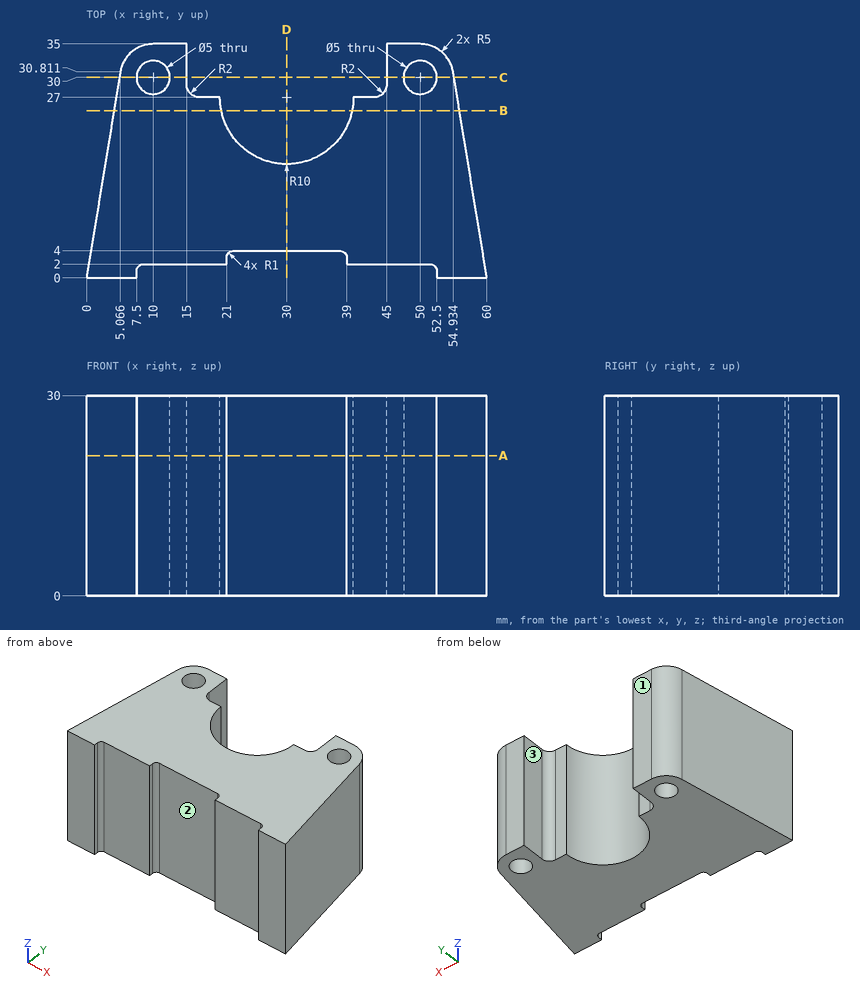
Job drawing, mm, ordinate dimensions from the low corner. One solid piece. A direction names the side the tool comes from. Round coordinates to 2 decimals unless told otherwise and drop trailing zeros. Loops run counter-clockwise (first coordinate to the right, second up) from the corner with the lowest first, then second, coordinate; pieces in that order, holes last. Notation, with made-up numbers: M 40,-29 L 91,-29 A7 cw 91,-16 Z; hole C 73.5,42.25 d11. An arc over 180 degrees is marked long. One line per question, with ' | ' between items. Start each with the question number.
Item 1: Cut at A-A, the plane z = 21. Write the cut outline in (x, y), plus the area to 3 significant figures.
Item 2: Wall check: line 1 (Y direction, x = 10, z = 19.75); line 2 (X direction, y = 24, z = 12); line 3 (X direction, y = 24.5, z = 5.25). Give the ranges that are in metal, low to high.
Item 3: Pin check, flat tips, straight feed: pin 1 Ø5 at (x, y) = (19.5, 5) entering from -Z; pin 2 Ø3.5 at (x, z) = (18, 19.5) entering from +Y; pin 3 Ø0.8 at (y, z) = (2.5, 21.5) entering from -X (1 decimal); pin 4 Ø6.5 at (y, z) = (31, 21) entering from +X. Stop position of each tip, or through.
Item 4: Which spindle directions (+Z, -Z, +X, -X, +Y, -Y) get a long thin tool onto all of the face, cutting with end or side? Do the marked faces 1, 2 and 3. Say none if no direction does.
Item 5: Cut at C-C, the plane y = 30. Write the cut outline in (x, z).
Item 6: Cut at B-B, the plane y = 25. Write the cut outline in (x, z).
Item 7: Cut at D-D, the plane x = 30. Write the cut outline in (y, z).
Responses:
1) outline: M 0,0 L 7.5,0 L 7.5,1 A1 cw 8.5,2 L 21,2 L 21,3 A1 cw 22,4 L 38,4 A1 cw 39,3 L 39,2 L 51.5,2 A1 cw 52.5,1 L 52.5,0 L 60,0 L 54.93,30.81 A5 ccw 50,35 L 45,35 L 45,29 A2 cw 43,27 L 40,27 A10 cw 20,27 L 17,27 A2 cw 15,29 L 15,35 L 10,35 A5 ccw 5.07,30.81 Z; hole C 10,30 d5; hole C 50,30 d5 | area: 1,330 mm²
2) line 1: y = 2 to 27.5, 32.5 to 35 | line 2: x = 3.95 to 20.46, 39.54 to 56.05 | line 3: x = 4.03 to 20.32, 39.68 to 55.97
3) pin 1: stops at z = 0 | pin 2: stops at y = 27.15 | pin 3: stops at x = 0.3 | pin 4: stops at x = 55.44
4) face 1: +Z, -Z, +X, -X, +Y | face 2: +Z, -Z, -Y | face 3: +Z, -Z, +Y
5) outline: M 4.93,0 L 7.5,0 L 7.5,30 L 4.93,30 Z; M 12.5,0 L 15,0 L 15,30 L 12.5,30 Z; M 45,0 L 47.5,0 L 47.5,30 L 45,30 Z; M 52.5,0 L 55.07,0 L 55.07,30 L 52.5,30 Z
6) outline: M 4.11,0 L 20.2,0 L 20.2,30 L 4.11,30 Z; M 39.8,0 L 55.89,0 L 55.89,30 L 39.8,30 Z
7) outline: M 4,0 L 17,0 L 17,30 L 4,30 Z
